The listing builds one solid part. Answer for the finished solid, in the listing's coordinates (mm). Round coordinates to 2 decimals unless told otherwise and drop trailing zeros. Order: outer loops, then holes, each group sorted by start corner. A loop starts at its lowest first (then second) coordinate and runs counter-clockwise, first axis right, second up. Notation, with made-up numbers: (88, 59) -> (108, 59) arc R30 ccw to (108, 93) -> close; hole circle Ø2 at (21.25, 9.5). An arc over 180 degrees is marked (long way). Return JSON: item names as keys, results as strings. Group by question number.
(1) Each of these flat-tipped pins is pushed along its axis until it touches: pin 1 (14.5 mm diameter, centred on x = 0, y = -6.83, fed in from +Z); pin 2 (1 mm diameter, centred on x = 72, z = 1, fed in from +Y); pin 3 (0.6 mm diameter, centred on y = 30.5, z = 1.5, fed in from +X); pin 4 (8 mm diameter, centred on x = 0, y = 32.53, fed in from -Z). Where does it stop, or does it pass through?
(2) The part is cut by section B-B (x = 0). Determine the outline of the cut face in (y, z).
(3) The part is cut by section A-A (y = -37). Determine the outline of the cut face in (x, z).
(4) The part is cut by section C-C (z = 0.9). Determine the outline of the cut face in (x, y), plus the area to 3 significant figures.
(5) Consider line 1 (Y direction, x = 0, z = 0.5); line 2 (X direction, y = -37, z = 1.1); line 3 (Y direction, x = -3, z = 1.2). Determine where each line is inside the solid, lowest interval first. Write a range as [from, to].
(6) Determine the mould class of faces 1 (the face through (73.097, -34.262, 1.014)), 2 (the face through (12, -11, 0)), 3 (the face through (-0.586, 36.987, 1.014)) for opening direction Y: +Y half, -Y half, draft (parallel to the pull), parting line (faces both ways), or undercut.
(7) The part is cut by section D-D (x = 54). Determine the outline of the cut face in (y, z), plus the area to 3 significant figures.
from build123d import *

# Parameters (mm, degrees)
SKETCH_1_W          = 36
SKETCH_1_H          = 110
EXTRUDE_1_DEPTH     = 2
SKETCH_2_W          = 110
SKETCH_2_H          = 36
EXTRUDE_2_DEPTH     = 2
SKETCH_3_R          = 4.5
CUT_EXTRUDE_1_DEPTH = 108.205410311


with BuildPart() as part:
    # 草图1 → 凸台-拉伸1 (new body)
    with BuildSketch(Plane.XY):
        Rectangle(SKETCH_1_W, SKETCH_1_H)
    extrude(amount=EXTRUDE_1_DEPTH)

    # 草图2 → 凸台-拉伸2 (add)
    with BuildSketch(Plane.XY.offset(2)):
        with Locations((37, -37)):
            Rectangle(SKETCH_2_W, SKETCH_2_H)
    extrude(amount=-EXTRUDE_2_DEPTH)

    # 草图3 → 切除-拉伸1 (cut, through all)
    with BuildSketch(Plane.XY.offset(2)):
        with Locations((0, 32.525719086)):
            Circle(SKETCH_3_R)
        with Locations((0, -6.833134262)):
            Circle(SKETCH_3_R)
        with Locations(Location((30.166865738, -37, 0), (0, 0, 180))):
            Circle(SKETCH_3_R)
        with Locations(Location((69.525719086, -37, 0), (0, 0, 180))):
            Circle(SKETCH_3_R)
    extrude(amount=-CUT_EXTRUDE_1_DEPTH, mode=Mode.SUBTRACT)


solid = part.part
Answer below:
{
 "1": {"pin 1": "stops at z = 2", "pin 2": "stops at y = -19", "pin 3": "stops at x = 18", "pin 4": "passes through"},
 "2": {"outline": "(-55, 0) -> (-11.33, 0) -> (-11.33, 2) -> (-55, 2) -> close; (-2.33, 0) -> (28.03, 0) -> (28.03, 2) -> (-2.33, 2) -> close; (37.03, 0) -> (55, 0) -> (55, 2) -> (37.03, 2) -> close"},
 "3": {"outline": "(-18, 0) -> (25.67, 0) -> (25.67, 2) -> (-18, 2) -> close; (34.67, 0) -> (65.03, 0) -> (65.03, 2) -> (34.67, 2) -> close; (74.03, 0) -> (92, 0) -> (92, 2) -> (74.03, 2) -> close"},
 "4": {"outline": "(-18, -55) -> (92, -55) -> (92, -19) -> (18, -19) -> (18, 55) -> (-18, 55) -> close; hole circle Ø9 at (0, -6.83); hole circle Ø9 at (0, 32.53); hole circle Ø9 at (30.17, -37); hole circle Ø9 at (69.53, -37)", "area": "6,370 mm²"},
 "5": {"line 1": "y = [-55, -11.33], [-2.33, 28.03], [37.03, 55]", "line 2": "x = [-18, 25.67], [34.67, 65.03], [74.03, 92]", "line 3": "y = [-55, -10.19], [-3.48, 29.17], [35.88, 55]"},
 "6": {"face 1": "undercut", "face 2": "draft", "face 3": "undercut"},
 "7": {"outline": "(-55, 0) -> (-19, 0) -> (-19, 2) -> (-55, 2) -> close", "area": "72.0 mm²"}
}
